Verification items for the finished model (mm, model axes). Face numbers are marked on the shaded views. A direction names the side the tool comes from. Coordinates: 2 decimals unless noted, no trailing zeros. Write each loop counter-clockwise with the first axis right and the second up, starting at its lowest first coordinate (ties: lowest second). Pieces come first, ordered by that corner, then holes. Notation, with made-up numbers: (-15, 15) -> (2, 15) arc R32 cw to (2, 46) -> close; hole circle Ø5 at (30.5, -26.5). An arc over 180 degrees is marked (long way). Answer in a Markdown table with one row per item.
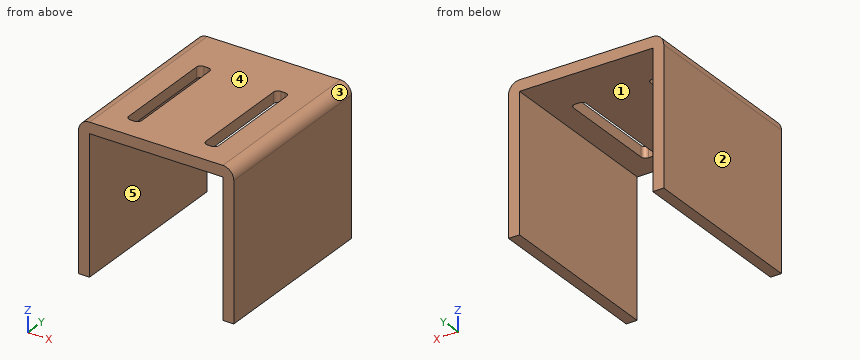
```python
from build123d import *

# Parameters (mm, degrees)
F1_DEPTH = 80
F3_DEPTH = 67.001


with BuildPart() as f1:
    # F0 (on Front) → F1 (new body)
    with BuildSketch(Plane.XZ):
        with BuildLine():
            Line((-35.25, 62), (-35.25, 0))
            Line((-35.25, 0), (-30.25, 0))
            Line((-30.25, 0), (-30.25, 62))
            Line((-30.25, 62), (30.25, 62))
            Line((30.25, 62), (30.25, 0))
            Line((30.25, 0), (35.25, 0))
            Line((35.25, 0), (35.25, 62))
            ThreePointArc((35.25, 62), (33.785534, 65.535534), (30.25, 67))
            Line((30.25, 67), (-30.25, 67))
            ThreePointArc((-30.25, 67), (-33.785534, 65.535534), (-35.25, 62))
        make_face()
    extrude(amount=-F1_DEPTH)

    # F2 (on face) → F3 (cut, through all)
    with BuildSketch(Plane.XY.offset(67)):
        with BuildLine():
            Line((16.534872, 10), (18.465128, 10))
            ThreePointArc((18.465128, 10), (19.879342, 10.585786), (20.465128, 12))
            Line((20.465128, 12), (20.465128, 58))
            ThreePointArc((20.465128, 58), (19.879342, 59.414214), (18.465128, 60))
            Line((18.465128, 60), (16.534872, 60))
            ThreePointArc((16.534872, 60), (15.120658, 59.414214), (14.534872, 58))
            Line((14.534872, 58), (14.534872, 12))
            ThreePointArc((14.534872, 12), (15.120658, 10.585786), (16.534872, 10))
        make_face()
        with BuildLine():
            Line((-18.465128, 10), (-16.534872, 10))
            ThreePointArc((-16.534872, 10), (-15.120658, 10.585786), (-14.534872, 12))
            Line((-14.534872, 12), (-14.534872, 58))
            ThreePointArc((-14.534872, 58), (-15.120658, 59.414214), (-16.534872, 60))
            Line((-16.534872, 60), (-18.465128, 60))
            ThreePointArc((-18.465128, 60), (-19.879342, 59.414214), (-20.465128, 58))
            Line((-20.465128, 58), (-20.465128, 12))
            ThreePointArc((-20.465128, 12), (-19.879342, 10.585786), (-18.465128, 10))
        make_face()
    extrude(amount=-F3_DEPTH, mode=Mode.SUBTRACT)


solid = f1.part
```
1. Access from +Z, -Z, +X, -X, +Y, -Y to the whole of each face (thin tool, end or side, straight path). Record for the marked faces 1 and 2.
Findings below:
| item | result |
|---|---|
| face 1 | -Z, +Y, -Y |
| face 2 | +Z, -Z, -X, +Y, -Y |
2. Sectioned sample at A-A, the plane z = 27. Record the cut outline in (x, y).
Findings below:
| item | result |
|---|---|
| outline | (-35.25, 0) -> (-30.25, 0) -> (-30.25, 80) -> (-35.25, 80) -> close; (30.25, 0) -> (35.25, 0) -> (35.25, 80) -> (30.25, 80) -> close |
3. Material ranges on probe 1 along X at (y, z) = (45, 26.5); probe 2 along Y at (x, z) = (18, 62.5); probe 3 along Z at (x, y) = (6.5, 13.5), recorded low to high. Write a range as from..to.
Findings below:
| item | result |
|---|---|
| probe 1 | x = -35.25..-30.25, 30.25..35.25 |
| probe 2 | y = 0..10, 60..80 |
| probe 3 | z = 62..67 |
4. Sectioned sample at C-C, the plane y = 67. Record the cut outline in (x, z).
Findings below:
| item | result |
|---|---|
| outline | (-35.25, 0) -> (-30.25, 0) -> (-30.25, 62) -> (30.25, 62) -> (30.25, 0) -> (35.25, 0) -> (35.25, 62) arc R5 ccw to (30.25, 67) -> (-30.25, 67) arc R5 ccw to (-35.25, 62) -> close |
5. Sectioned sample at B-B, the plane y = 24.5. Record the cut outline in (x, z), and give its area (3 significant figures).
Findings below:
| item | result |
|---|---|
| outline | (-35.25, 0) -> (-30.25, 0) -> (-30.25, 62) -> (-20.47, 62) -> (-20.47, 67) -> (-30.25, 67) arc R5 ccw to (-35.25, 62) -> close; (-14.53, 62) -> (14.53, 62) -> (14.53, 67) -> (-14.53, 67) -> close; (20.47, 62) -> (30.25, 62) -> (30.25, 0) -> (35.25, 0) -> (35.25, 62) arc R5 ccw to (30.25, 67) -> (20.47, 67) -> close |
| area | 902 mm² |
6. Go/stop test with flat-tipped pins: pin 1 (2 mm diameter, centred on x = -7, y = 13.5, fed in from -Z); pin 2 (2.5 mm diameter, centred on y = 31, z = 64, fed in from +X); pin 3 (2.5 mm diameter, centred on y = 28, z = 64, fed in from -X). Record where each tip stops, or that it passes through.
Findings below:
| item | result |
|---|---|
| pin 1 | stops at z = 62 |
| pin 2 | stops at x = 35.19 |
| pin 3 | stops at x = -35.19 |
7. Release check for a two-part mould opening along X. For the marked faces 3, 4 and 5 record: released by +X, released by -X, zero draft, split by the parting line, or undercut.
Findings below:
| item | result |
|---|---|
| face 3 | released by +X |
| face 4 | zero draft |
| face 5 | undercut |
8. Sectioned sample at D-D, the plane x = -26. Record the cut outline in (y, z), and give its area (3 significant figures).
Findings below:
| item | result |
|---|---|
| outline | (0, 62) -> (80, 62) -> (80, 67) -> (0, 67) -> close |
| area | 400 mm² |
